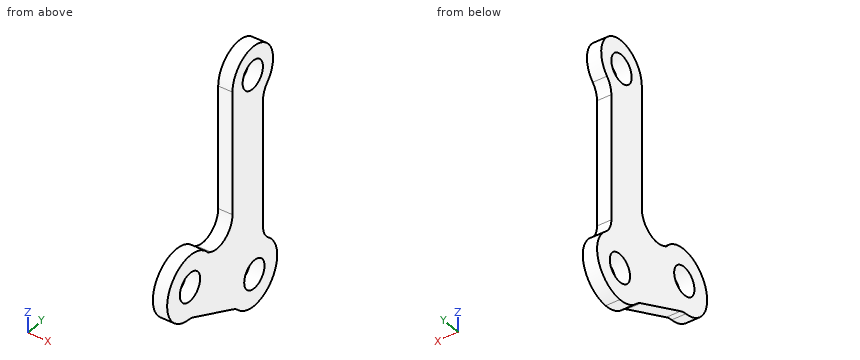
```python
from build123d import *

# Parameters (mm, degrees)
EXTRUDE_1_DEPTH     = 2
SKETCH_1_3_R        = 2
CUT_EXTRUDE_1_DEPTH = 35.66133887
FILLET_1_R          = 3


with BuildPart() as part:
    # 草图1 → 凸台-拉伸1 (new body)
    with BuildSketch(Plane(origin=(0, 0, 0), x_dir=(0, 0, -1), z_dir=(1, 0, 0))):
        with BuildLine():
            Line((-25, -6), (-25, 0))
            Line((-25, 0), (-21.535898385, 0))
            ThreePointArc((-21.535898385, 0), (-28.464101615, 0), (-25, -6))
        make_face()
        with BuildLine():
            Line((-21.535898385, 0), (-25, 0))
            Line((-25, 0), (-25, -6))
            ThreePointArc((-25, -6), (-22.171572875, -4.828427125), (-21, -2))
            ThreePointArc((-21, -2), (-21.136296695, -0.96472382), (-21.535898385, 0))
        make_face()
        with BuildLine():
            Line((-0.545176611, 0), (-21.535898385, 0))
            ThreePointArc((-21.535898385, 0), (-21.136296695, -0.96472382), (-21, -2))
            ThreePointArc((-21, -2), (-22.171572875, -4.828427125), (-25, -6))
            Line((-25, -6), (-2.797845949, -6))
            Line((-2.797845949, -6), (-0.871249866, -1.868401368))
            ThreePointArc((-0.871249866, -1.868401368), (-0.807766841, -0.916826597), (-0.545176611, 0))
        make_face()
        with BuildLine():
            ThreePointArc((8.125231148, -1.690473047), (4.486383017, 2.726360373), (-0.545176611, 0))
            Line((-0.545176611, 0), (0, 0))
            Line((0, 0), (7.250462296, -3.380946094))
            Line((7.250462296, -3.380946094), (6.37921243, -5.249347462))
            ThreePointArc((6.37921243, -5.249347462), (7.66521356, -3.67252807), (8.125231148, -1.690473047))
        make_face()
        with BuildLine():
            Line((0, 0), (-0.545176611, 0))
            ThreePointArc((-0.545176611, 0), (-0.807766841, -0.916826597), (-0.871249866, -1.868401368))
            Line((-0.871249866, -1.868401368), (0, 0))
        make_face()
        with BuildLine():
            Line((-0.871249866, -1.868401368), (-2.797845949, -6))
            Line((-2.797845949, -6), (0, -6))
            Line((0, -6), (0, -4.356499889))
            ThreePointArc((0, -4.356499889), (-0.621910323, -3.177681615), (-0.871249866, -1.868401368))
        make_face()
        with BuildLine():
            Line((0, -6), (-2.797845949, -6))
            Line((-2.797845949, -6), (-5.045405798, -10.819907651))
            ThreePointArc((-5.045405798, -10.819907651), (-0.389642338, -10.300397024), (2.205056498, -14.200853745))
            Line((2.205056498, -14.200853745), (6.37921243, -5.249347462))
            ThreePointArc((6.37921243, -5.249347462), (3.001481776, -6.147034134), (0, -4.356499889))
            Line((0, -4.356499889), (0, -6))
        make_face()
        with BuildLine():
            Line((7.250462296, -3.380946094), (0, 0))
            Line((0, 0), (0, -4.356499889))
            ThreePointArc((0, -4.356499889), (3.001481776, -6.147034134), (6.37921243, -5.249347462))
            Line((6.37921243, -5.249347462), (7.250462296, -3.380946094))
        make_face()
        with BuildLine():
            Line((0, -4.356499889), (0, 0))
            Line((0, 0), (-0.871249866, -1.868401368))
            ThreePointArc((-0.871249866, -1.868401368), (-0.621910323, -3.177681615), (0, -4.356499889))
        make_face()
        with BuildLine():
            ThreePointArc((2.205056498, -14.200853745), (-0.389642338, -10.300397024), (-5.045405798, -10.819907651))
            Line((-5.045405798, -10.819907651), (-5.916655664, -12.688309019))
            Line((-5.916655664, -12.688309019), (1.333806632, -16.069255112))
            Line((1.333806632, -16.069255112), (2.205056498, -14.200853745))
        make_face()
        with BuildLine():
            Line((-5.916655664, -12.688309019), (-5.045405798, -10.819907651))
            ThreePointArc((-5.045405798, -10.819907651), (-4.27347954, -18.418764477), (2.208575484, -14.378782065))
            ThreePointArc((2.208575484, -14.378782065), (2.207695651, -14.289800508), (2.205056498, -14.200853745))
            Line((2.205056498, -14.200853745), (1.333806632, -16.069255112))
            Line((1.333806632, -16.069255112), (-5.916655664, -12.688309019))
        make_face()
    extrude(amount=EXTRUDE_1_DEPTH)

    # 草图1<3> → 切除-拉伸1 (cut, through all)
    with BuildSketch(Plane(origin=(0, 0, 0), x_dir=(0, 0, -1), z_dir=(1, 0, 0))):
        with Locations((-25, -2)):
            Circle(SKETCH_1_3_R)
        with Locations((3.625231148, -1.690473047)):
            Circle(SKETCH_1_3_R)
        with Locations((-2.291424516, -14.378782065)):
            Circle(SKETCH_1_3_R)
    extrude(amount=CUT_EXTRUDE_1_DEPTH, mode=Mode.SUBTRACT)

    # 圆角1
    fillet_1_edges = [part.edges().sort_by_distance(p)[0] for p in [
        (1, -6, 2.797845949),
        (1, 0, 0.545176611),
        (1, -5.249347462, -6.37921243),
        (1, -14.200853745, -2.205056498),
        (1, 0, 21.535898385),
    ]]
    fillet(fillet_1_edges, radius=FILLET_1_R)


solid = part.part
```
CAD build for the part. Positions are in the model's coordinates, mm. Give positions to 0.01 mm unless a question says otherwise; leave off trailing zeros. Write each loop counter-clockwise with the first axis right and the second up, starting at its lowest first coordinate (ties: lowest second). Pieces come first, ordered by that corner, then holes. Notation, with made-up numbers: M 39,54 L 55,54 A26 ccw 55,76 Z; hole C 78,-39.5 d5. An arc over 180 degrees is marked long. Return JSON: item names as keys, results as strings. Group by question number.
(1) Band-saw the part on B-B (y = -13.25). Give the cut face in (x, z).
(2) Band-saw the part on D-D (z = 16). Give the cut face in (x, y).
(3) Band-saw the part on C-C (x = 1.45). State how many separate pieces and enclosed holes the cut face has, and give its area (3 significant figures).
(4) Flat gauge pin, fed straight in: pin 1 Ø1 at (y, z) = (-7.5, 20.5) entering from +X. Where does the tip first touch, or does it go through?
(5) Band-saw the part on A-A (z = 24.5). Give the cut face in (x, y).
(6) Drill centre lines: L1, parallel to Z at x = 0.75, y = -1.5; L2, parallel to Z at x = 0.55, y = -2; L3, parallel to Y at x = 0.75, z = 25. Where is each one in solid material? Low to high. Write a range as [from, to].
Entries:
{
 "1": {"outline": "M 0,-2.65 L 2,-2.65 L 2,0.64 L 0,0.64 Z; M 0,3.94 L 2,3.94 L 2,6.65 L 0,6.65 Z"},
 "2": {"outline": "M 0,-6 L 2,-6 L 2,0 L 0,0 Z"},
 "3": {"separate pieces": "1", "enclosed holes": "3", "area": "317 mm^2"},
 "4": {"pin 1": "passes through"},
 "5": {"outline": "M 0,-6 L 2,-6 L 2,-3.94 L 0,-3.94 Z; M 0,-0.06 L 2,-0.06 L 2,1.97 L 0,1.97 Z"},
 "6": {"L1": "z = [-8.12, -5.62], [-1.63, 23.06], [26.94, 28.97]", "L2": "z = [-8.11, -5.6], [-1.65, 23], [27, 29]", "L3": "y = [-6, -4], [0, 2]"}
}
